Design review of the part shown in the three views and the two pictorial views. Dimensions are in mm from the part's minimum x, y and z. Give positions to 0.01 mm unless a question says otherwise; leave off trailing zeros. Order: outer loops, then holes, each group sorted by start corner. A loop starts at its lowest first (then second) coordinate and runs counter-clockwise, first axis right, second up.
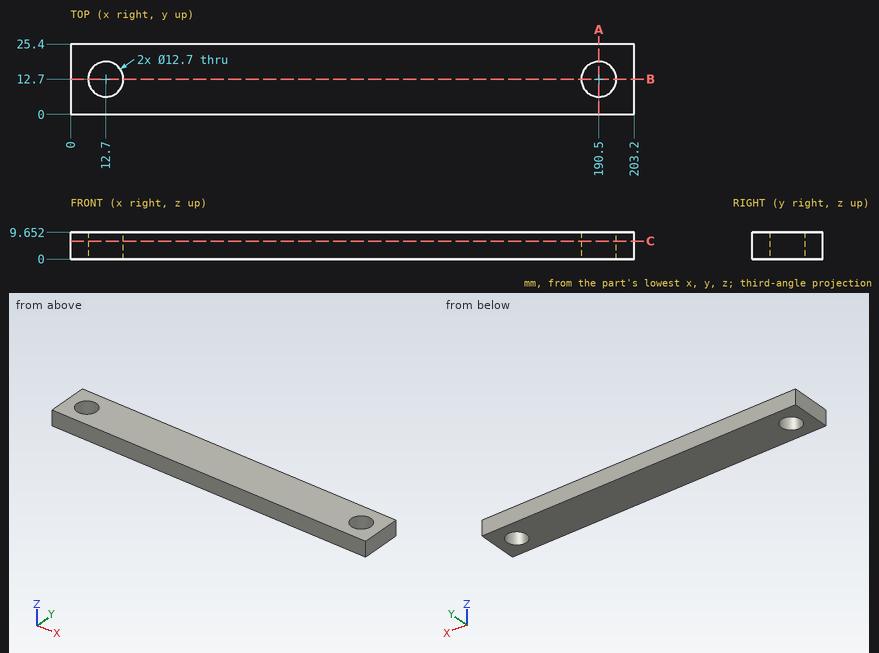
Item 1: Take a section at A-A (x = 190.5). Give the boundary of the cut face in (y, z).
Values found:
outline: (0, 0) - (6.35, 0) - (6.35, 9.65) - (0, 9.65) - close; (19.05, 0) - (25.4, 0) - (25.4, 9.65) - (19.05, 9.65) - close
Item 2: For line 1 (X direction, y = 10.75, z = 8); line 2 (Y direction, x = 190.5, z = 3); line 3 (X direction, y = 15.5, z = 2.25), list the stretches that pass through material, from the lowest coordinate up.
Values found:
line 1: x = 0 to 6.66, 18.74 to 184.46, 196.54 to 203.2
line 2: y = 0 to 6.35, 19.05 to 25.4
line 3: x = 0 to 7, 18.4 to 184.8, 196.2 to 203.2
Item 3: Take a section at B-B (y = 12.7). Give the boundary of the cut face in (x, z), and give its area (3 significant figures).
Values found:
outline: (0, 0) - (6.35, 0) - (6.35, 9.65) - (0, 9.65) - close; (19.05, 0) - (184.15, 0) - (184.15, 9.65) - (19.05, 9.65) - close; (196.85, 0) - (203.2, 0) - (203.2, 9.65) - (196.85, 9.65) - close
area: 1,720 mm2
Item 4: Take a section at C-C (z = 6.5). Give the boundary of the cut face in (x, y), and give its area (3 significant figures).
Values found:
outline: (0, 0) - (203.2, 0) - (203.2, 25.4) - (0, 25.4) - close; hole circle Ø12.7 at (12.7, 12.7); hole circle Ø12.7 at (190.5, 12.7)
area: 4,910 mm2
